from build123d import *

# Parameters (mm, degrees)
F0_R     = 2
F1_DEPTH = 1


with BuildPart() as f1:
    # F0 (on Top) → F1 (new body)
    with BuildSketch(Plane.XY):
        with BuildLine():
            Line((-35, 15), (-35, 0))
            Line((-35, 0), (-6, 0))
            Line((-6, 0), (-6, -2))
            ThreePointArc((-6, -2), (-4.242641, -6.242641), (0, -8))
            Line((0, -8), (3.9375, -8))
            Line((3.9375, -8), (10.5, -18))
            Line((10.5, -18), (13, -18))
            Line((13, -18), (13, -11))
            Line((13, -11), (20.116628, -11))
            Line((20.116628, -11), (20.116628, -5.116628))
            Line((20.116628, -5.116628), (0, 15))
            Line((0, 15), (-35, 15))
        make_face()
        with Locations((0, -2)):
            Circle(F0_R, mode=Mode.SUBTRACT)
    extrude(amount=F1_DEPTH)


solid = f1.part
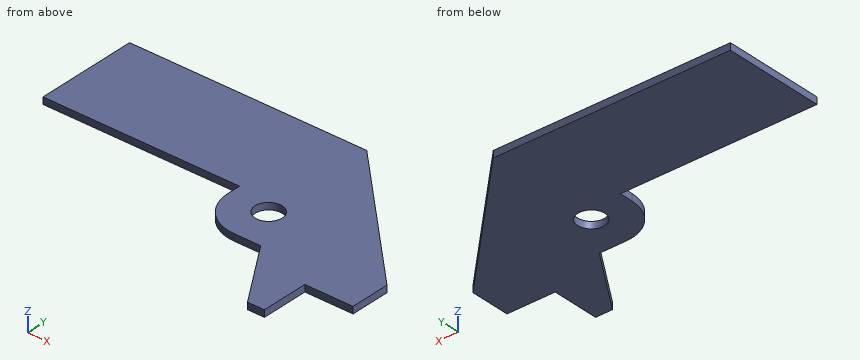
Build history of the part. All positions in model axes, mm. Give positions to 0.01 mm unless a question says otherwise; leave off trailing zeros. Order: outer loops, then holes, each group sorted by start corner. A loop starts at its lowest first (then second) coordinate and runs counter-clockwise, first axis right, second up. Notation, with made-up numbers: M -38.75,38.5 L -12.75,38.5 A16 cw -12.75,45.5 Z; hole C -4,37 d1. An arc over 180 degrees is marked long. Use one line per item in the form item = value.
Q1. Wall check: probe 1 along Y at (x, z) = (0, 0.7); probe 2 along Y at (x, z) = (-23, 0.5); probe 3 along Y at (x, z) = (-1.5, 0.1). Give the ranges that are in metal, low to high.
Conclusion:
probe_1 = -8 to -4, 0 to 15
probe_2 = 0 to 15
probe_3 = -7.81 to -3.32, -0.68 to 15
Q2. Pin check, flat tips, straight feed: P1, Ø0.5, axis at x = 16, z = 0.5, coming from the -Y side; P2, Ø0.5, axis at x = 2, z = 0.5, coming from the -Y side. Stop position of each tip, or through.
Conclusion:
P1 = -11
P2 = -8
Q3. Slice it at B-B, the plane y = 1. Write the cut outline in (x, z).
Conclusion:
outline = M -35,0 L 14,0 L 14,1 L -35,1 Z
Q4. Slice it at A-A, the plane z = 0.75. Write the cut outline in (x, y), and give its area (3 significant figures).
Conclusion:
outline = M -35,0 L -6,0 L -6,-2 A6 ccw 0,-8 L 3.94,-8 L 10.5,-18 L 13,-18 L 13,-11 L 20.12,-11 L 20.12,-5.12 L 0,15 L -35,15 Z; hole C 0,-2 d4
area = 892 mm2
Q5. Slice it at C-C, the plane x = -25.5. Write the cut outline in (y, z).
Conclusion:
outline = M 0,0 L 15,0 L 15,1 L 0,1 Z
